```python
from build123d import *

# Parameters (mm, degrees)
BOSS_EXTRUDE1_DEPTH      = 9.398
BOSS_EXTRUDE1_DEPTH_BACK = 9.398
SKETCH1_R                = 4.064


with BuildPart() as part:
    # Sketch1 → Boss-Extrude1 (new, two sides: drawn at the far end of the back side and taken through both)
    with BuildSketch(Plane(origin=(0, 0, 0), x_dir=(0, 0, -1), z_dir=(1, 0, 0)).offset(-BOSS_EXTRUDE1_DEPTH_BACK)):
        Circle(SKETCH1_R)
    extrude(amount=BOSS_EXTRUDE1_DEPTH + BOSS_EXTRUDE1_DEPTH_BACK)

    # Sketch5 → Revolve1 (revolve)
    with BuildSketch(Plane(origin=(0, 0, 0), x_dir=(1, 0, 0), z_dir=(0, 1, 0))):
        with BuildLine():
            Line((9.398, 0), (9.398, 4.318))
            add(Edge.make_bspline(
                [(9.398, 4.318), (10.668, 2.595439575), (10.668, 0)],
                knots=[0, 0, 0, 1, 1, 1], degree=2))
            Line((10.668, 0), (9.398, 0))
        make_face()
    revolve1 = revolve(axis=Axis((9.398, 0, 0), (1, 0, 0)))

    # Mirror1: Revolve1 across plane
    add(revolve1.mirror(Plane(origin=(0, 0, 0), x_dir=(0, 0, 1), z_dir=(1, 0, 0))))


solid = part.part
```
Source: CAD feature listing. Evaluate the final solid. Frame: model axes, mm. Round coordinates to 2 decimals unless told otherwise and drop trailing zeros. Write each loop counter-clockwise with the first axis right and the second up, starting at its lowest first coordinate (ties: lowest second). Pieces come first, ordered by that corner, then holes. Notation, with made-up numbers: M 68.5,69 L 127.5,69 A15 cw 127.5,83 Z; hole C 42,-9 d8. An arc over 180 degrees is marked long. Answer as a JSON object with one key per item and string values. Group by question number.
(1) Section query A-A on x = 5.25. Output: boundary loops of the cut face in (y, z).
(2) First-contact query: pin 1 (2.5 mm diameter, centred on y = 0, z = 1, fed in from +X); pin 2 (3 mm diameter, centred on y = 3.5, z = 1, fed in from -X); pin 3 (3 mm diameter, centred on y = -1, z = 3, fed in from -X); pin 4 (1.5 mm diameter, centred on x = 1.5, y = 1.5, fed in from -Z). Flat tips, straight axial feed; report the tip coordinate or a pass-through.
(3) Ray query, line 1 (Y direction, x = 7.5, z = 0); line 2 (X direction, y = 2.75, z = 2.25); line 3 (X direction, y = -1.5, z = 2.5). Return the intervals inside material, ascending. Write a range as [from, to].
Computed values:
{
 "1": {"outline": "C 0,0 d8.13"},
 "2": {"pin 1": "x = 10.67", "pin 2": "x = -10.42", "pin 3": "x = -10.52", "pin 4": "z = -3.99"},
 "3": {"line 1": "[-4.06, 4.06]", "line 2": "[-9.88, 9.88]", "line 3": "[-10.17, 10.17]"}
}
